The listing builds one solid part. Answer for the finished solid, in the listing's coordinates (mm). A direction names the side the tool comes from. Give positions to 0.01 mm unless a question says otherwise; leave off trailing zeros. Loops run counter-clockwise (first coordinate to the right, second up) from the corner with the lowest first, then second, coordinate; pieces in that order, holes last. Notation, with made-up numbers: M 74,82.25 L 78,82.25 A12 ccw 78,86.25 Z; hole C 41,-16.5 d1. An arc over 180 degrees is marked long. Return JSON: item names as keys, results as strings.
from build123d import *

# Parameters (mm, degrees)
SKETCH1_R           = 2.2
BOSS_EXTRUDE1_DEPTH = 10
FILLET1_R           = 6.35
FILLET2_R           = 6.35
FILLET3_R           = 0.5


with BuildPart() as part:
    # Sketch1 → Boss-Extrude1 (new body)
    with BuildSketch(Plane(origin=(0, 0, 0), x_dir=(1, 0, 0), z_dir=(0, 1, 0))):
        Polygon((127, 0), (-127, 0), (-127, -50.8), (-114.3, -50.8), (-114.3, -25.4), (-107.95, -19.05), (107.95, -19.05), (114.3, -25.4), (114.3, -50.8), (127, -50.8), align=None)
        with Locations(Location((-120.65, -6.35, 0), (0, 0, 270))):
            Circle(SKETCH1_R, mode=Mode.SUBTRACT)
        with Locations(Location((-107.95, -6.35, 0), (0, 0, 270))):
            Circle(SKETCH1_R, mode=Mode.SUBTRACT)
        with Locations(Location((-120.65, -44.45, 0), (0, 0, 270))):
            Circle(SKETCH1_R, mode=Mode.SUBTRACT)
        with Locations(Location((120.65, -44.45, 0), (0, 0, 90))):
            Circle(SKETCH1_R, mode=Mode.SUBTRACT)
        with Locations(Location((107.95, -6.35, 0), (0, 0, 90))):
            Circle(SKETCH1_R, mode=Mode.SUBTRACT)
        with Locations(Location((120.65, -6.35, 0), (0, 0, 90))):
            Circle(SKETCH1_R, mode=Mode.SUBTRACT)
    extrude(amount=BOSS_EXTRUDE1_DEPTH)

    # Fillet1
    fillet1_edges = [part.edges().sort_by_distance(p)[0] for p in [
        (127, 5, 0),
        (127, 5, 50.8),
        (114.3, 5, 50.8),
        (-114.3, 5, 50.8),
        (-127, 5, 50.8),
        (-127, 5, 0),
    ]]
    fillet(fillet1_edges, radius=FILLET1_R - 0.0001)  # a hair under: the kernel refuses the full size

    # Fillet2
    fillet2_edges = [part.edges().sort_by_distance(p)[0] for p in [
        (114.3, 5, 25.4),
        (107.95, 5, 19.05),
        (-107.95, 5, 19.05),
        (-114.3, 5, 25.4),
    ]]
    fillet(fillet2_edges, radius=FILLET2_R)

    # Fillet3
    fillet3_edges = [part.edges().sort_by_distance(p)[0] for p in [
        (0, 0, 0),
        (0, 10, 0),
        (-127, 0, 25.4),
        (127, 0, 25.4),
        (-114.3, 0, 36.240178061),
        (-125.14015735, 0, 1.85984265),
        (-125.14015735, 0, 48.94015735),
        (-116.15984265, 0, 48.94015735),
        (116.15984265, 0, 48.94015735),
        (125.14015735, 0, 48.94015735),
        (125.14015735, 0, 1.85984265),
        (127, 10, 25.4),
        (-127, 10, 25.4),
        (-114.3, 10, 36.240178061),
        (-125.14015735, 10, 1.85984265),
        (-125.14015735, 10, 48.94015735),
        (-116.15984265, 10, 48.94015735),
        (116.15984265, 10, 48.94015735),
        (125.14015735, 10, 48.94015735),
        (125.14015735, 10, 1.85984265),
        (114.3, 0, 36.240178061),
        (114.3, 10, 36.240178061),
        (111.125, 0, 22.225),
        (111.125, 10, 22.225),
        (0, 0, 19.05),
        (0, 10, 19.05),
        (-111.125, 0, 22.225),
        (-111.125, 10, 22.225),
        (113.816635031, 0, 25.600216326),
        (113.816635031, 10, 25.600216326),
        (107.749783674, 0, 19.533364969),
        (107.749783674, 10, 19.533364969),
        (-113.816635031, 0, 25.600216326),
        (-113.816635031, 10, 25.600216326),
        (-107.749783674, 0, 19.533364969),
        (-107.749783674, 10, 19.533364969),
    ]]
    fillet(fillet3_edges, radius=FILLET3_R)


solid = part.part
(1) A tool of negligible diameter and unlimited length cuts with its end or side. For faces 4 (the flat face through (-2, 0, 8)), 5 (the flat face through (114.3, 5, 36)), from which of +Z, -Z, +X, -X, +Y, -Y can it reach the whole face along a straight path? Write none if from no direction.
Values follow:
{"face 4": "+Z, -Z, +X, -X, -Y", "face 5": "+Z, +Y, -Y"}
(2) Determine the mould class of faces 1 (the cylindrical face through (125.19, 5.06, 48.89)), 2 (the cylindrical face through (-107.782, 5.063, 19.547)), 3 (the flat face through (2, 5, 0)) for opening direction X: released by +X, released by -X, zero draft, split by the parting line, or undercut.
Values follow:
{"face 1": "released by +X", "face 2": "undercut", "face 3": "zero draft"}
(3) Straight lines are drawn through the part: line 1 along X through (y, z) = (2.5, 44.45); line 2 along X through (y, z) = (4, 6.35); line 3 along X through (y, z) = (1.75, 33). For each, find the intervals that lie inside material, in ascending order.
Values follow:
{"line 1": "-127 to -122.85, -118.45 to -114.3, 114.3 to 118.45, 122.85 to 127", "line 2": "-127 to -122.85, -118.45 to -110.15, -105.75 to 105.75, 110.15 to 118.45, 122.85 to 127", "line 3": "-127 to -114.3, 114.3 to 127"}
(4) The part is cut by section B-B (x = -52). Determine the outline of the cut face in (y, z), and give its area (3 significant figures).
Values follow:
{"outline": "M 0,0.5 A0.5 ccw 0.5,0 L 9.5,0 A0.5 ccw 10,0.5 L 10,18.55 A0.5 ccw 9.5,19.05 L 0.5,19.05 A0.5 ccw 0,18.55 Z", "area": "190 mm²"}
(5) Given pin 1 (1.5 mm diameter, centred on x = -95.5, y = 8, fed in from +Z), flat-ended and moving along its own axis, determine where the tip first touches the part or whether it passes through.
Values follow:
{"pin 1": "z = 19.05"}
(6) The part is cut by section A-A (y = 5). Give the number of separate pieces and of enclosed holes in the cut face, and give its area (3 significant figures).
Values follow:
{"separate pieces": "1", "enclosed holes": "6", "area": "5,550 mm²"}
